Input: dimensioned drawing with shaded views. Units: mm. Origin: part minimum x, y, z. Coordinates: 2 decimals unless noted, no trailing zeros. Loops run counter-clockwise (first coordinate to the right, second up) from the corner with the lowest first, then second, coordinate; pieces in that order, holes last.
Item 1: Section B-B on y = 4. Return loops of the section in (x, z) (1 decimal).
Item 2: Section D-D on y = 7. Return loops of the section in (x, z).
Item 3: Section C-C on z = 1.7. Return loops of the section in (x, y).
Item 4: Contact query for flat-ended pins moving along their axis: P1, Ø0.7, axis at x = 1, y = 8, coming from the +Z side; P2, Ø0.7, axis at y = 7.5, z = 1, coming from the -X side; P3, Ø0.7, axis at x = 1.5, y = 2, coming from the -Z side. Output: stop coordinate, or through.
Item 5: Ray query, line 1 along Y through (x, z) = (1.6, 0.85); line 2 along Y through (x, z) = (2.3, 2.1); line 3 along X through (y, z) = (9.5, 1.5). Return the intervals inside material, ascending.
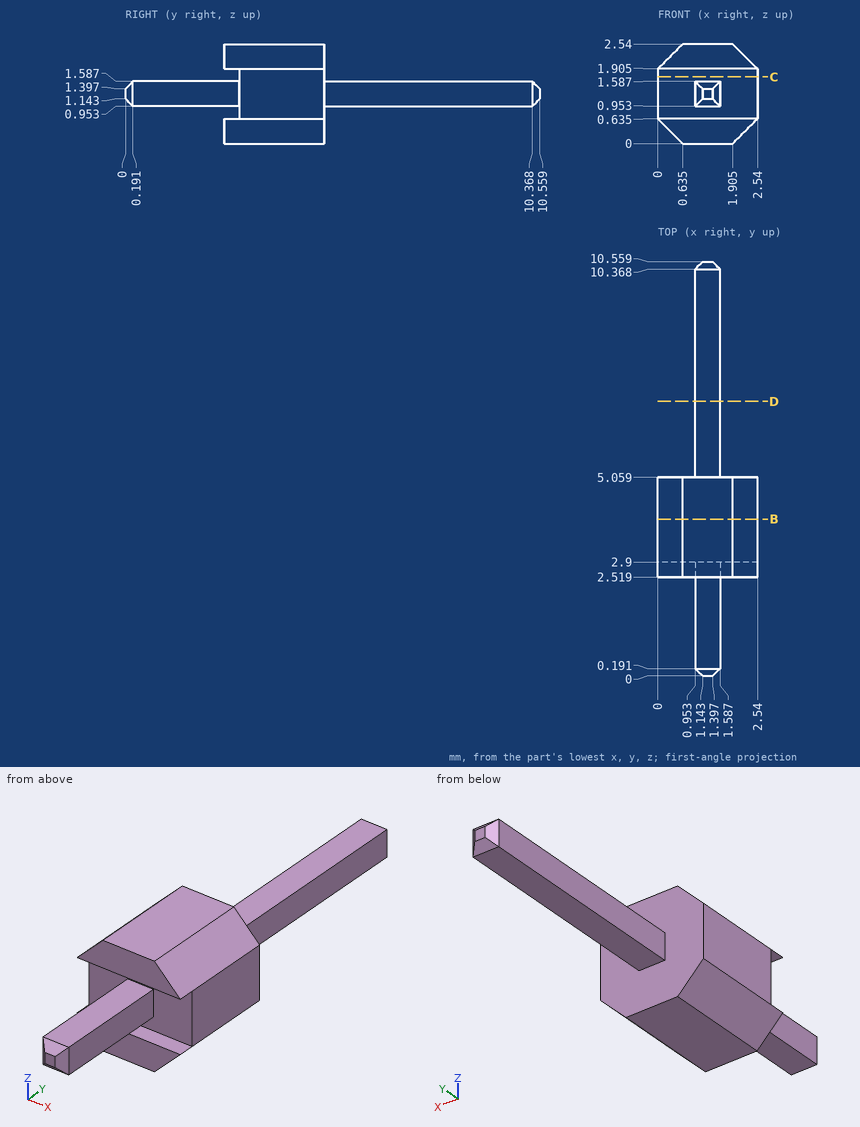
Results found:
1. outline: (0, 0.6) - (0.6, 0) - (1.9, 0) - (2.5, 0.6) - (2.5, 1.9) - (1.9, 2.5) - (0.6, 2.5) - (0, 1.9) - close
2. outline: (0.95, 0.95) - (1.59, 0.95) - (1.59, 1.59) - (0.95, 1.59) - close
3. outline: (0, 2.9) - (2.54, 2.9) - (2.54, 5.06) - (0, 5.06) - close
4. P1: stops at z = 1.59
4. P2: stops at x = 0.95
4. P3: stops at z = 0.95
5. line 1: y = 2.9 to 5.06
5. line 2: y = 2.52 to 5.06
5. line 3: x = 0.95 to 1.59
